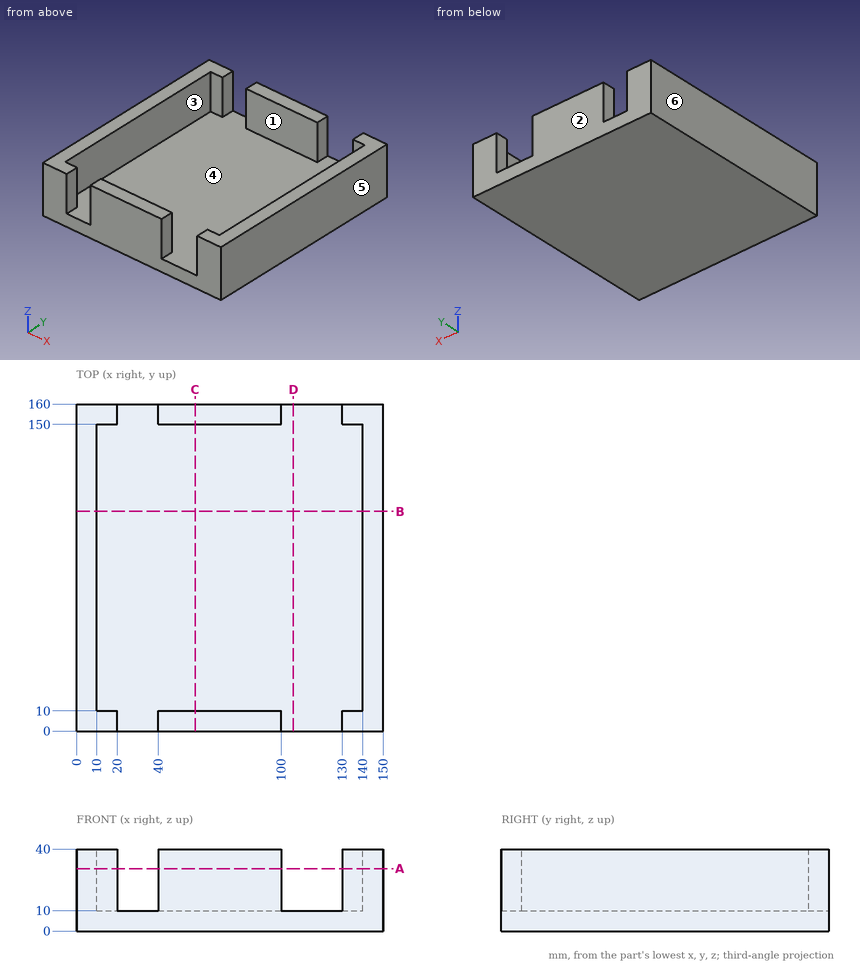
Source: three-view drawing plus pictorial views. Frame: mm from the lowest corner of the part. A direction names the side the tool comes from. Coordinates: 2 decimals unless noted, no trailing zeros. Loops run counter-clockwise (first coordinate to the right, second up) from the corner with the lowest first, then second, coordinate; pieces in that order, holes last. Notation, with made-up numbers: (-2, 21) -> (3, 21) arc R18 ccw to (3, 39) -> close; hole circle Ø10 at (69.25, 44.5). An arc over 180 degrees is marked (long way). Answer in a Markdown table with one row per item. Add a question column.
Q1. Section C-C on x = 58. Return the cut outline in (y, z), and give its area (3 significant figures).
Q2. Reachability of the marked faces 1 and 2 from +Z, -Z, +X, -X, +Y, -Y: full face, straight path, thin tool, end or side. Return the list, or none.
Q3. Section D-D on x = 106. Return the cut outline in (y, z).
Q4. Ray query, line 1 along X through (y, z) = (87.5, 30); line 2 along Y through (x, z) = (48, 29); line 3 along Z through (x, y) = (118, 134). Return the intervals inside material, ascending.
Q5. Section A-A on z = 30.5. Return the cut outline in (x, y).
Q6. Contact query for flat-ended pins moving along their axis: pin 1 Ø1 at (x, y) = (127.5, 134.5) entering from +Z; pin 2 Ø12 at (y, z) = (55, 15) entering from -X. Output: stop coordinate, or through.
Q7. Pull-direction query (X, two-part tool) for the marked faces 3, 4, 5 and 6; classes: pulls with the +X half, pulls with the -X half, needs draft (parallel to the pull), parting line crosses it, or undercut.
Q8. Section B-B on y = 107.5. Return the cut outline in (x, z).
Computed values:
| question | item | result |
|---|---|---|
| 1 | outline | (0, 0) -> (160, 0) -> (160, 40) -> (150, 40) -> (150, 10) -> (10, 10) -> (10, 40) -> (0, 40) -> close |
| 1 | area | 2,200 mm^2 |
| 2 | face 1 | +Z |
| 2 | face 2 | +Z, -Z, +X, -X, +Y |
| 3 | outline | (0, 0) -> (160, 0) -> (160, 10) -> (0, 10) -> close |
| 4 | line 1 | x = 0 to 10, 140 to 150 |
| 4 | line 2 | y = 0 to 10, 150 to 160 |
| 4 | line 3 | z = 0 to 10 |
| 5 | outline | (0, 0) -> (20, 0) -> (20, 10) -> (10, 10) -> (10, 150) -> (20, 150) -> (20, 160) -> (0, 160) -> close; (40, 0) -> (100, 0) -> (100, 10) -> (40, 10) -> close; (40, 150) -> (100, 150) -> (100, 160) -> (40, 160) -> close; (130, 0) -> (150, 0) -> (150, 160) -> (130, 160) -> (130, 150) -> (140, 150) -> (140, 10) -> (130, 10) -> close |
| 6 | pin 1 | stops at z = 10 |
| 6 | pin 2 | stops at x = 0 |
| 7 | face 3 | undercut |
| 7 | face 4 | undercut |
| 7 | face 5 | pulls with the +X half |
| 7 | face 6 | pulls with the -X half |
| 8 | outline | (0, 0) -> (150, 0) -> (150, 40) -> (140, 40) -> (140, 10) -> (10, 10) -> (10, 40) -> (0, 40) -> close |
